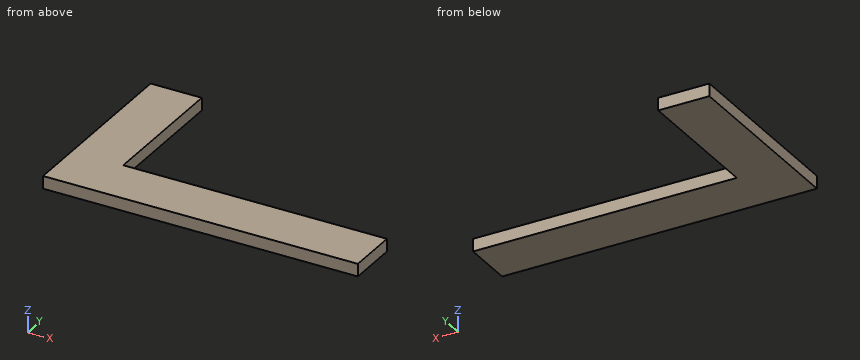
Autodesk Fusion 360 part; units mm, degrees
sketch "スケッチ1" plane through (0, 0, 0) normal (0, 0, 1) x (1, 0, 0)
  line L0 (0, 0) -> (250, 0)
  line L1 (250, 0) -> (250, 150)
  line L2 (250, 150) -> (0, 150)
  line L3 (0, 150) -> (0, 0)
  line L4 (250, 150) -> (40.6, 150)
  line L5 (40.6, 150) -> (40.6, 40.6)
  line L6 (40.6, 40.6) -> (250, 40.6)
  line L7 (250, 40.6) -> (250, 150)
  dimension "d1" = 250
  dimension "d2" = 150
  dimension "d3" = 40.6
  dimension "d4" = 40.6
extrude "押し出し1" add sketch "スケッチ1" along normal blind 10 contours L0 L1 L2 L3 L5 L6
Design review of the part built by this model. Coordinates are the model's own, in mm. Round coordinates to 2 decimals unless told otherwise and drop trailing zeros. Write each loop counter-clockwise with the first axis right and the second up, starting at its lowest first coordinate (ties: lowest second). Pieces come first, ordered by that corner, then holes. Notation, with made-up numbers: (70, 36) -> (95, 36) arc R29 cw to (95, 56) -> close; hole circle Ø3 at (52, 76.5). An arc over 180 degrees is marked (long way). One line per question, with ' | ' between items.
(1) Insertion check: P1, Ø4, axis at y = 132, z = 5.5, coming from the +X side; P2, Ø2, axis at x = 105.5, z = 2.5, coming from the +Y side. Each pin has a flat end and moves straight along its axis. Give the tip position at first contact, or say it passes through.
Result sheet:
P1: x = 40.6 | P2: y = 40.6
(2) Take a section at A-A, the plane z = 2.5. State the section outline as (x, y) points.
Result sheet:
outline: (0, 0) -> (250, 0) -> (250, 40.6) -> (40.6, 40.6) -> (40.6, 150) -> (0, 150) -> close
(3) Wall thickness on line 1 (Y direction, x = 209, z = 3.5): over which ranges is the line inside the solid? List them lowest first. Write a range as [from, to].
Result sheet:
line 1: [0, 40.6]
(4) Take a section at B-B, the plane y = 82. State the section outline as (x, z) points, and give its area (3 significant figures).
Result sheet:
outline: (0, 0) -> (40.6, 0) -> (40.6, 10) -> (0, 10) -> close | area: 406 mm2
